```python
from build123d import *

# Parameters (mm, degrees)
BOSS_EXTRUDE1_DEPTH                          = 7.5
SKETCH2_R                                    = 5
CUT_EXTRUDE1_DEPTH                           = 45.237992721
SKETCH3_W                                    = 2
SKETCH3_H                                    = 19
CUT_EXTRUDE2_DEPTH                           = 45.237992721
CBORE_FOR_SOCKET_HEAD_CAP_SCREW1_D           = 6.6
CBORE_FOR_SOCKET_HEAD_CAP_SCREW1_DEPTH       = 11
CBORE_FOR_SOCKET_HEAD_CAP_SCREW1_CBORE_D     = 11
CBORE_FOR_SOCKET_HEAD_CAP_SCREW1_CBORE_DEPTH = 6.5
TAPPED_HOLE1_D                               = 5
DIAMETER_HOLE1_D                             = 6.6


with BuildPart() as part:
    # Sketch1 → Boss-Extrude1 (new, symmetric)
    with BuildSketch(Plane.XY):
        Polygon((-24, 0), (24, 0), (24, 6), (12, 6), (12, 34), (-12, 34), (-12, 6), (-24, 6), align=None)
    extrude(amount=BOSS_EXTRUDE1_DEPTH, both=True)

    # Sketch2 → Cut-Extrude1 (cut, through all)
    with BuildSketch(Plane.XY.offset(7.5)):
        with Locations((0, 15)):
            Circle(SKETCH2_R)
    extrude(amount=-CUT_EXTRUDE1_DEPTH, mode=Mode.SUBTRACT)

    # Sketch3 → Cut-Extrude2 (cut, through all)
    with BuildSketch(Plane.XY.offset(7.5)):
        with Locations((0, 24.5)):
            Rectangle(SKETCH3_W, SKETCH3_H)
    extrude(amount=-CUT_EXTRUDE2_DEPTH, mode=Mode.SUBTRACT)

    # CBORE for Socket Head Cap Screw1
    with Locations(Plane(origin=(12, 0, 0), x_dir=(0, 0, -1), z_dir=(1, 0, 0))):
        with Locations((0, 27)):
            CounterBoreHole(CBORE_FOR_SOCKET_HEAD_CAP_SCREW1_D / 2, CBORE_FOR_SOCKET_HEAD_CAP_SCREW1_CBORE_D / 2, CBORE_FOR_SOCKET_HEAD_CAP_SCREW1_CBORE_DEPTH, depth=CBORE_FOR_SOCKET_HEAD_CAP_SCREW1_DEPTH)

    # Tapped Hole1 (through all)
    with Locations(Plane(origin=(-1, 0, 0), x_dir=(0, 0, -1), z_dir=(1, 0, 0))):
        with Locations((0, 27)):
            Hole(TAPPED_HOLE1_D / 2)

    # Diameter Hole1 (through all)
    with Locations(Plane(origin=(0, 6, 0), x_dir=(1, 0, 0), z_dir=(0, 1, 0))):
        with Locations((18, 0), (-18, 0)):
            Hole(DIAMETER_HOLE1_D / 2)


solid = part.part
```
For this review, take the finished solid that the model builds, in its own axes (mm). A direction names the side the tool comes from. Give positions to 0.01 mm unless a question says otherwise; leave off trailing zeros. Write each loop counter-clockwise with the first axis right and the second up, starting at its lowest first coordinate (ties: lowest second). Pieces come first, ordered by that corner, then holes. Notation, with made-up numbers: M -17,-4 L -13,-4 A10 ccw -13,10 Z; hole C 73,-0.5 d2. An arc over 180 degrees is marked long. Answer as a JSON object with one key per item and string values. Group by question number.
Item 1: Consider section B-B on x = -18. Write out the cut boundary in (y, z).
Item 2: Consider section D-D on x = -6.5. Write out the cut boundary in (y, z).
Item 3: Tool access review of faces 1 (the flat face through (-19.2, 6, 3.4)), 2 (the flat face through (-24, 3, 0)), 3 (the flat face through (16.8, 6, 3.4)), 4 (the cylindrical face through (3.22, 23.78, -0.72)), 5 (the flat face through (-1, 30, 0)): name each direction out of +Z, -Z, +X, -X, +Y, -Y from which nothing blocks a thin tool from reaching the whole face with its end or side.
Item 4: For probe 1 along Y at (x, z) = (7.25, 0); probe 2 along X at (y, z) = (23.5, -5.5); probe 3 along Y at (x, z) = (-7.5, 0), list the stretches that pass through material, from the lowest coordinate up. Write a range as [from, to].
Item 5: Consider section A-A on y = 27. Write out the cut boundary in (x, z).
Item 6: For pin 1 Ø7.5 at (y, z) = (22.5, -1.5) entering from -X; pin 2 Ø16 at (x, y) = (0, 15) entering from +Z; pin 3 Ø3.5 at (x, z) = (-16.5, 3) entering from +Y; pin 4 Ø3.5 at (y, z) = (27.5, -2) entering from +X, all flat-tipped, find the tip position at first contact; note any pin that passes through.
Item 7: Consider section C-C on z = 0. Count the separate pieces of the cut face and the enclosed holes in it, plus the area to 3 significant figures.
Item 8: Draft analysis for pull direction Z (two halves, no side actions). For faces 6 (the flat face through (1, 24, 2)), 7 (the cylindrical face through (-6.58, 29.48, -0.33)), 8 (the flat face through (-0.3, 9.7, -7.5)), state which applies: +Z half, -Z half, draft (parallel to the pull), parting line (faces both ways), or undercut.
Check result:
{
 "1": {"outline": "M 0,-7.5 L 6,-7.5 L 6,-3.3 L 0,-3.3 Z; M 0,3.3 L 6,3.3 L 6,7.5 L 0,7.5 Z"},
 "2": {"outline": "M 0,-7.5 L 34,-7.5 L 34,7.5 L 0,7.5 Z; hole C 27,0 d5"},
 "3": {"face 1": "+Z, -Z, -X, +Y", "face 2": "+Z, -Z, -X, +Y, -Y", "face 3": "+Z, -Z, +X, +Y", "face 4": "+X", "face 5": "+Z, -Z, +Y"},
 "4": {"probe 1": "y = [0, 21.5], [32.5, 34]", "probe 2": "x = [-12, -1], [1, 12]", "probe 3": "y = [0, 24.5], [29.5, 34]"},
 "5": {"outline": "M -12,-7.5 L -1,-7.5 L -1,-2.5 L -12,-2.5 Z; M -12,2.5 L -1,2.5 L -1,7.5 L -12,7.5 Z; M 1,-7.5 L 12,-7.5 L 12,-5.5 L 5.5,-5.5 L 5.5,-3.3 L 1,-3.3 Z; M 1,3.3 L 5.5,3.3 L 5.5,5.5 L 12,5.5 L 12,7.5 L 1,7.5 Z"},
 "6": {"pin 1": "stops at x = -12", "pin 2": "stops at z = 7.5", "pin 3": "stops at y = 6", "pin 4": "stops at x = 5.5"},
 "7": {"separate pieces": "5", "enclosed holes": "0", "area": "618 mm^2"},
 "8": {"face 6": "draft", "face 7": "undercut", "face 8": "-Z half"}
}
